Drawing for the job (mm, zero at the part's lowest x, y, z). A direction names the side the tool comes from. Round coordinates to 2 decimals unless told otherwise and drop trailing zeros. Write each loop counter-clockwise with the first axis right and the second up, starting at its lowest first coordinate (ties: lowest second). Pieces come first, ordered by that corner, then holes.
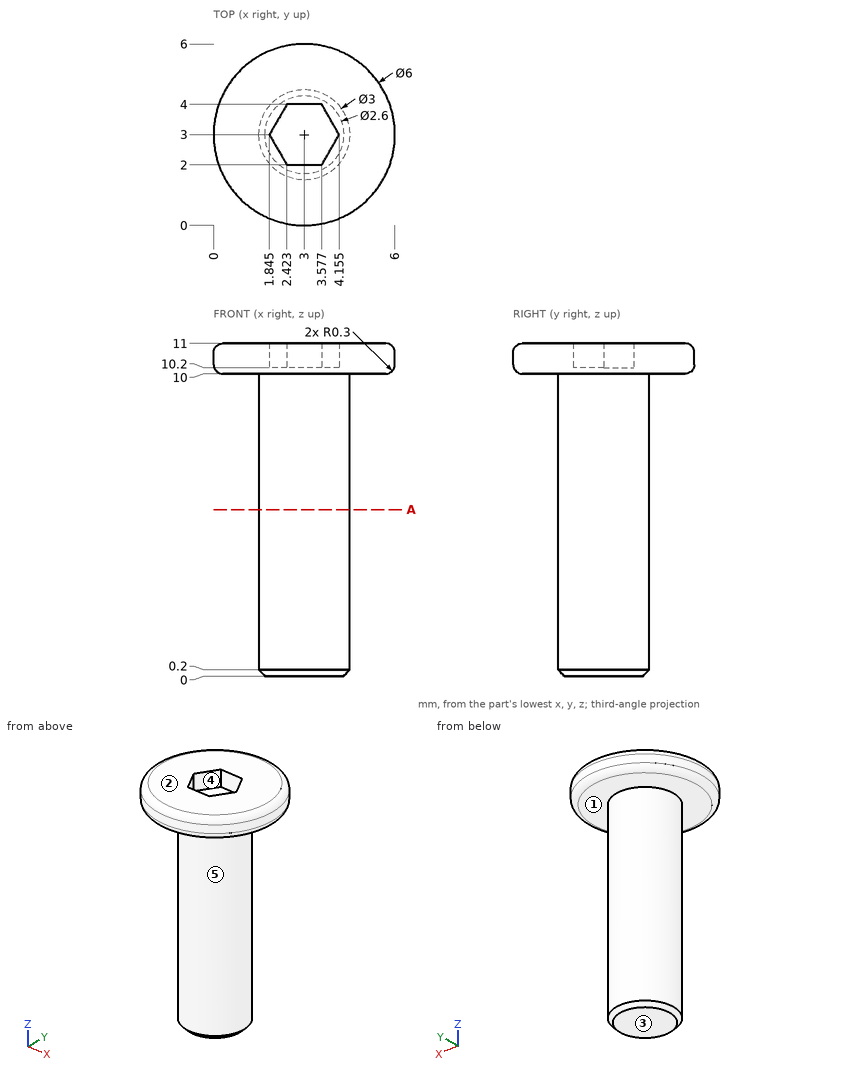
1) Wall check: probe 1 along X at (y, z) = (2.25, 6); probe 2 along Z at (x, y) = (0.75, 2.75); probe 3 along Y at (x, z) = (3.5, 7) (1 decimal). Give the ranges that are in metal, low to high.
2) Flat gauge pins, fed straight in: pin 1 Ø1 at (x, z) = (2, 3) entering from +Y; pin 2 Ø1.5 at (y, z) = (1.5, 2.5) entering from -X. Where does each tip first touch, or does it go through?
3) Cut at A-A on z = 5.5. List the corners of the cut face in (x, y).
4) Pull direction X, two halves, no side cores. Call the marked faces 3, 4 and 5: released by +X, released by -X, zero draft, split by the parting line, or undercut.
5) Which spindle directions (+Z, -Z, +X, -X, +Y, -Y) get a long thin tool onto all of the face, cutting with end or side? Do the marked faces 1 and 2. Say none if no direction does.
Result sheet:
1. probe 1: x = 1.7 to 4.3
1. probe 2: z = 10 to 11
1. probe 3: y = 1.6 to 4.4
2. pin 1: stops at y = 4.41
2. pin 2: stops at x = 1.7
3. outline: circle Ø3 at (3, 3)
4. face 3: zero draft
4. face 4: undercut
4. face 5: split by the parting line
5. face 1: -Z
5. face 2: +Z, +X, -X, +Y, -Y
